```python
from build123d import *

# Parameters (mm, degrees)
F1_DEPTH = 15
F3_DEPTH = 5
F5_DEPTH = 8
F8_D     = 5
F9_D     = 5


with BuildPart() as f1:
    # F0 (on Top) → F1 (new body)
    with BuildSketch(Plane.XY):
        with BuildLine():
            Line((20, -52.3067873225), (20, -62.8967407741))
            ThreePointArc((20, -62.8967407741), (0, 66), (-20, -62.8967407741))
            Line((-20, -62.8967407741), (-20, -52.3067873225))
            ThreePointArc((-20, -52.3067873225), (0, 56), (20, -52.3067873225))
        make_face()
    extrude(amount=F1_DEPTH)

    # F2 (on Top) → F3 (join)
    with BuildSketch(Plane.XY):
        with BuildLine():
            Line((20, 0), (20, -52.3067873225))
            ThreePointArc((20, -52.3067873225), (0, 56), (-20, -52.3067873225))
            Line((-20, -52.3067873225), (-20, 0))
            ThreePointArc((-20, 0), (0, 20), (20, 0))
        make_face()
    extrude(amount=F3_DEPTH)

    # F4 (on face) → F5 (cut)
    with BuildSketch(Plane.XY.offset(15)):
        with BuildLine():
            ThreePointArc((20, -62.8967407741), (49.6744428377, -43.4562967677), (64.9973116988, -11.460779726))
            Line((64.9973116988, -11.460779726), (55.1492341687, -9.7242979493))
            ThreePointArc((55.1492341687, -9.7242979493), (43.1876018012, -35.6487173775), (20, -52.3067873225))
            Line((20, -52.3067873225), (20, -62.8967407741))
        make_face()
        with BuildLine():
            Line((-64.9973116988, 11.460779726), (-55.1492341687, 9.7242979493))
            ThreePointArc((-55.1492341687, 9.7242979493), (0, 56), (55.1492341687, 9.7242979493))
            Line((55.1492341687, 9.7242979493), (64.9973116988, 11.460779726))
            ThreePointArc((64.9973116988, 11.460779726), (0, 66), (-64.9973116988, 11.460779726))
        make_face()
        with BuildLine():
            ThreePointArc((-20, -62.8967407741), (0, -66), (20, -62.8967407741))
            Line((20, -62.8967407741), (20, -52.3067873225))
            ThreePointArc((20, -52.3067873225), (0, -56), (-20, -52.3067873225))
            Line((-20, -52.3067873225), (-20, -62.8967407741))
        make_face()
        with BuildLine():
            ThreePointArc((-64.9973116988, -11.460779726), (-49.6744428377, -43.4562967677), (-20, -62.8967407741))
            Line((-20, -62.8967407741), (-20, -52.3067873225))
            ThreePointArc((-20, -52.3067873225), (-43.1876018012, -35.6487173775), (-55.1492341687, -9.7242979493))
            Line((-55.1492341687, -9.7242979493), (-64.9973116988, -11.460779726))
        make_face()
    extrude(amount=-F5_DEPTH, mode=Mode.SUBTRACT)

    # F8 (through all)
    with Locations(Plane(origin=(0, 0, 0), x_dir=(1, 0, 0), z_dir=(0, 0, -1))):
        with Locations((43.13, 43.13), (43.1370270186, -43.13), (-43.13, 41.36), (-43.1229729814, -44.9)):
            Hole(F8_D / 2)

    # F9 (through all)
    with Locations(Plane.XY.offset(5)):
        with Locations((30, -30), (30, 30), (-30, 31.8642704598), (-30, -28.1357295402)):
            Hole(F9_D / 2)


solid = f1.part
```
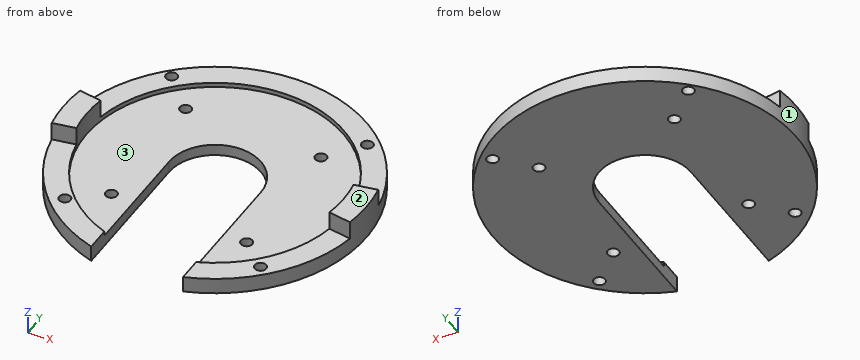
Work out the finished part from the listing and answer in its coordinate system (mm). Face numbers are marked on the shaded views. Coordinates: 2 decimals unless noted, no trailing zeros. Loops run counter-clockwise (first coordinate to the right, second up) from the corner with the lowest first, then second, coordinate; pieces in that order, holes last. Notation, with made-up numbers: (-14.5, -6) -> (4.5, -6) arc R26 ccw to (4.5, 25) -> close; hole circle Ø3 at (-30, 17.5). An arc over 180 degrees is marked (long way). Answer as CSV lines item,"result".
Q1. The part is cut by section B-B on x = -43.13. Write down the section's boundary in (y, z), and give its area (3 significant figures).
Findings:
outline,"(-49.96, 0) -> (-43.86, 0) -> (-43.86, 7) -> (-49.96, 7) -> close; (-38.86, 0) -> (42.4, 0) -> (42.4, 7) -> (35.72, 7) -> (35.72, 5) -> (-35.72, 5) -> (-35.72, 7) -> (-38.86, 7) -> close; (47.4, 0) -> (49.96, 0) -> (49.96, 7) -> (47.4, 7) -> close"
area,"487 mm²"
Q2. Each of these flat-tipped pins is pushed along its axis until it touches: pin 1 (3.5 mm diameter, centred on y = -17.5, z = 3, fed in from +X); pin 2 (2 mm diameter, centred on x = 32, z = 6.5, fed in from -Y); pin 3 (7.5 mm diameter, centred on y = -22.5, z = 5, fed in from -X). Where does it stop, or does it pass through?
Findings:
pin 1,"stops at x = 64.09"
pin 2,"stops at y = -58.27"
pin 3,"stops at x = -63.28"
Q3. The part is cut by section D-D on x = 0. Write down the section's boundary in (y, z), and give its area (3 significant figures).
Findings:
outline,"(20, 0) -> (66, 0) -> (66, 7) -> (56, 7) -> (56, 5) -> (20, 5) -> close"
area,"250 mm²"
Q4. The part is cut by section C-C on y = 5.5. Write down the section's boundary in (x, z).
Findings:
outline,"(-65.77, 0) -> (-19.23, 0) -> (-19.23, 5) -> (-55.73, 5) -> (-55.73, 15) -> (-65.77, 15) -> close; (19.23, 0) -> (65.77, 0) -> (65.77, 15) -> (55.73, 15) -> (55.73, 5) -> (19.23, 5) -> close"
Q5. Find the intervals of material crossed by probe 1 along X at (y, z) = (-41.36, 3.5); probe 2 along X at (y, z) = (-43, 5.25); probe 3 along Y at (x, z) = (30, 3.45), in increasing order.
Findings:
probe 1,"x = -51.43 to -45.63, -40.63 to -20, 20 to 41.36, 44.9 to 51.43"
probe 2,"x = -50.07 to -45.02, -41.24 to -35.87, 35.87 to 40.63, 45.63 to 50.07"
probe 3,"y = -58.79 to -32.5, -27.5 to 27.5, 32.5 to 58.79"
Q6. The part is cut by section A-A on z = 8.5. Write down the section's boundary in (x, y), and give its area (3 significant figures).
Findings:
outline,"(-65, -11.46) -> (-55.15, -9.72) arc R56 cw to (-55.15, 9.72) -> (-65, 11.46) arc R66 ccw to start; (55.15, -9.72) -> (65, -11.46) arc R66 ccw to (65, 11.46) -> (55.15, 9.72) arc R56 cw to start"
area,"426 mm²"
Q7. For a pull along X with two mould halves and no side action, classify the marked faces 1, 2 and 3 as +X half, -X half, draft (parallel to the pull), parting line (faces both ways), or undercut.
Findings:
face 1,"parting line"
face 2,"draft"
face 3,"undercut"
